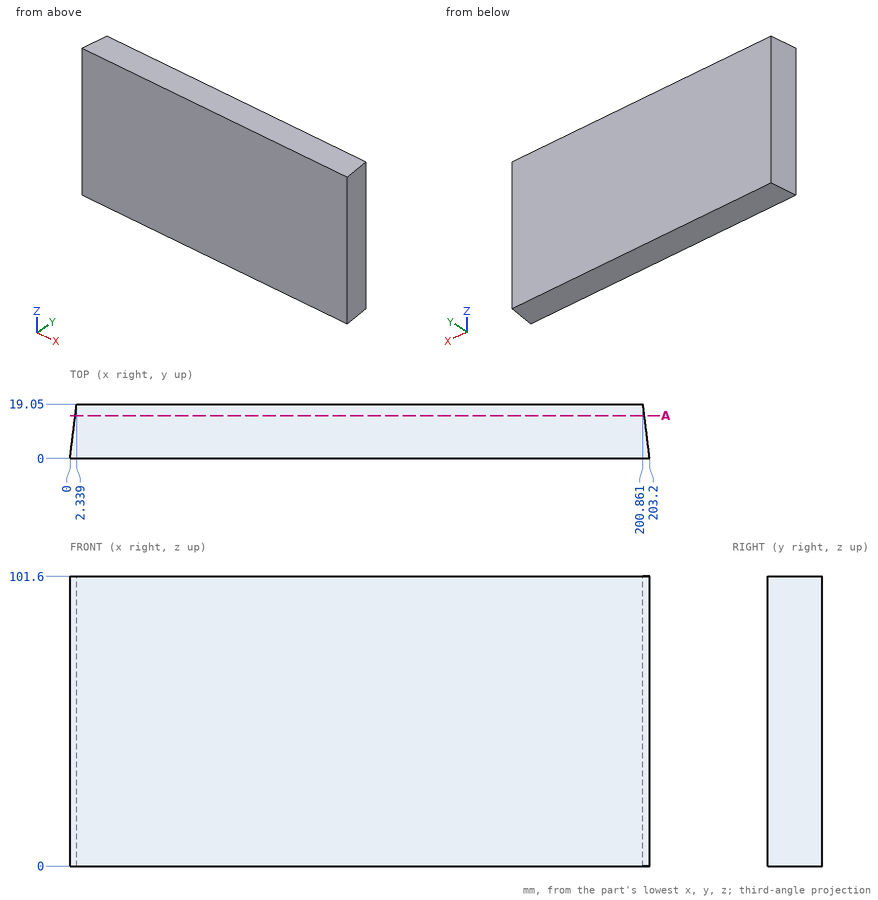
Answer from the drawing. Dimensions are ordinates in mm from the lowest x, y and z of the part. Give positions to 0.01 mm unless a question says otherwise; leave off trailing zeros. Loops run counter-clockwise (first coordinate to the right, second up) from the corner with the lowest first, then second, coordinate; pieces in that order, holes last. Notation, with made-up numbers: M 52,36.5 L 92,36.5 A28 cw 92,65.5 Z; hole C 64,49 d5. An arc over 180 degrees is marked long. One line per item, written item: value.
Q1. Find the intervals of material crossed by line 1 (X direction, y = 2.25, z = 6); line 2 (X direction, y = 12.75, z = 52.5), in increasing order. Write a range as from..to.
Working result:
line 1: x = 0.28..202.92
line 2: x = 1.57..201.63
Q2. A flat-ended cylindrical pin translates along its axis: P1, Ø2, axis at y = 2.5, z = 54.5, coming from the +X side. Find the tip coordinate at first contact, or state that the pin passes through.
Working result:
P1: stops at x = 203.02
Q3. A cutting plane is placed at A-A on y = 15. Determine the outline of the cut face in (x, z), then the cut area to 3 significant figures.
Working result:
outline: M 1.84,0 L 201.36,0 L 201.36,101.6 L 1.84,101.6 Z
area: 20,300 mm^2
